Verification items for the finished model (mm, model axes). Face numbers are marked on the shaded views. A direction names the side the tool comes from. Round coordinates to 2 decimals unless told otherwise and drop trailing zeros. Loops run counter-clockwise (first coordinate to the right, second up) from the corner with the lowest first, then second, coordinate; pieces in that order, holes last. Notation, with made-up numbers: (39.5, 80) -> (57.5, 80) arc R11 ccw to (57.5, 91) -> close; hole circle Ø8 at (-29, 84.25). An arc over 180 degrees is marked (long way). Use a Markdown table: item, result. Add a question column.
```python
from build123d import *

# Parameters (mm, degrees)
SKETCH1_W               = 58
SKETCH1_H               = 86
BOSS_EXTRUDE1_DEPTH     = 23
CUT_EXTRUDE1_DEPTH      = 23
CUT_EXTRUDE2_DEPTH      = 23
FILLET1_R               = 3
FILLET2_R               = 2
FILLET3_R               = 2
FILLET4_R               = 1
FILLET5_R               = 3
FILLET6_R               = 3
FILLET7_R               = 3
FILLET8_R               = 3
FILLET9_R               = 3
FILLET10_R              = 3
CUT_EXTRUDE3_DEPTH      = 57.73623181
CUT_EXTRUDE3_DEPTH_BACK = 57.73623181
SKETCH4_W               = 46
SKETCH4_H               = 18
CUT_EXTRUDE4_DEPTH      = 57.73623181
CUT_EXTRUDE4_DEPTH_BACK = 57.73623181
SKETCH5_R               = 2
SKETCH5_R_2             = 1.5
SKETCH6_R               = 1.5
CUT_EXTRUDE11_DEPTH     = 10
SKETCH7_R               = 1.5
CUT_EXTRUDE12_DEPTH     = 10


with BuildPart() as part:
    # Sketch1 → Boss-Extrude1 (new body)
    with BuildSketch(Plane(origin=(0, 0, 0), x_dir=(1, 0, 0), z_dir=(0, 1, 0))):
        Rectangle(SKETCH1_W, SKETCH1_H)
    extrude(amount=BOSS_EXTRUDE1_DEPTH)

    # Sketch2 → Cut-Extrude1 (cut)
    with BuildSketch(Plane(origin=(0, 0, 0), x_dir=(1, 0, 0), z_dir=(0, 1, 0))):
        Polygon((29, -23), (17, -23), (17, -17), (23, -17), (23, -7), (29, -7), align=None)
    extrude(amount=CUT_EXTRUDE1_DEPTH, mode=Mode.SUBTRACT)

    # Sketch3 → Cut-Extrude2 (cut)
    with BuildSketch(Plane(origin=(0, 0, 0), x_dir=(1, 0, 0), z_dir=(0, 1, 0))):
        Polygon((-15, -13), (-15, 22), (18, 22), (18, -1), (6, -1), (6, -13), align=None)
    extrude(amount=CUT_EXTRUDE2_DEPTH, mode=Mode.SUBTRACT)

    # Fillet1
    fillet1_edges = [part.edges().sort_by_distance(p)[0] for p in [
        (23, 11.5, 7),
    ]]
    fillet(fillet1_edges, radius=FILLET1_R)

    # Fillet2
    fillet2_edges = [part.edges().sort_by_distance(p)[0] for p in [
        (17, 11.5, 17),
    ]]
    fillet(fillet2_edges, radius=FILLET2_R)

    # Fillet3
    fillet3_edges = [part.edges().sort_by_distance(p)[0] for p in [
        (17, 11.5, 23),
    ]]
    fillet(fillet3_edges, radius=FILLET3_R)

    # Fillet4
    fillet4_edges = [part.edges().sort_by_distance(p)[0] for p in [
        (23, 11.5, 17),
    ]]
    fillet(fillet4_edges, radius=FILLET4_R)

    # Fillet5
    fillet5_edges = [part.edges().sort_by_distance(p)[0] for p in [
        (-15, 11.5, 13),
    ]]
    fillet(fillet5_edges, radius=FILLET5_R)

    # Fillet6
    fillet6_edges = [part.edges().sort_by_distance(p)[0] for p in [
        (6, 11.5, 13),
    ]]
    fillet(fillet6_edges, radius=FILLET6_R)

    # Fillet7
    fillet7_edges = [part.edges().sort_by_distance(p)[0] for p in [
        (-15, 11.5, -22),
    ]]
    fillet(fillet7_edges, radius=FILLET7_R)

    # Fillet8
    fillet8_edges = [part.edges().sort_by_distance(p)[0] for p in [
        (18, 11.5, -22),
    ]]
    fillet(fillet8_edges, radius=FILLET8_R)

    # Fillet9
    fillet9_edges = [part.edges().sort_by_distance(p)[0] for p in [
        (18, 11.5, 1),
    ]]
    fillet(fillet9_edges, radius=FILLET9_R)

    # Fillet10
    fillet10_edges = [part.edges().sort_by_distance(p)[0] for p in [
        (6, 11.5, 1),
    ]]
    fillet(fillet10_edges, radius=FILLET10_R)

    # Sketch4 → Cut-Extrude3 (cut, two sides: drawn at the far end of the back side and taken through both)
    with BuildSketch(Plane(origin=(0, 0, 0), x_dir=(0, 0, -1), z_dir=(1, 0, 0)).offset(-CUT_EXTRUDE3_DEPTH_BACK)):
        with Locations((0, 9)):
            Rectangle(SKETCH4_W, SKETCH4_H)
    extrude(amount=CUT_EXTRUDE3_DEPTH + CUT_EXTRUDE3_DEPTH_BACK, mode=Mode.SUBTRACT)

    # Sketch5 → Cut-Extrude4 (cut, two sides: drawn at the far end of the back side and taken through both)
    with BuildSketch(Plane(origin=(0, 0, 0), x_dir=(1, 0, 0), z_dir=(0, 1, 0)).offset(-CUT_EXTRUDE4_DEPTH_BACK)):
        with Locations(Location((20.5, -4, 0), (0, 0, 270))):
            Circle(SKETCH5_R)
        with Locations(Location((-20.5, -4, 0), (0, 0, 270))):
            Circle(SKETCH5_R)
        with Locations(Location((20, -14.5, 0), (0, 0, 270))):
            Circle(SKETCH5_R_2)
        with Locations(Location((-16.5, -38, 0), (0, 0, 270))):
            Circle(SKETCH5_R_2)
        with Locations(Location((25.5, -38, 0), (0, 0, 270))):
            Circle(SKETCH5_R_2)
        with Locations(Location((-24.051636808, -28.259079953, 0), (0, 0, 270))):
            Circle(SKETCH5_R_2)
    extrude(amount=CUT_EXTRUDE4_DEPTH + CUT_EXTRUDE4_DEPTH_BACK, mode=Mode.SUBTRACT)

    # Sketch6 → Cut-Extrude11 (cut)
    with BuildSketch(Plane.ZY.offset(29)):
        with Locations((40, 3)):
            Circle(SKETCH6_R)
        with Locations((26, 18)):
            Circle(SKETCH6_R)
    extrude(amount=-CUT_EXTRUDE11_DEPTH, mode=Mode.SUBTRACT)

    # Sketch7 → Cut-Extrude12 (cut)
    with BuildSketch(Plane(origin=(0, 0, -43), x_dir=(-1, 0, 0), z_dir=(0, 0, -1))):
        with Locations((-19.5, 4.5)):
            Circle(SKETCH7_R)
        with Locations((-19.5, 18.5)):
            Circle(SKETCH7_R)
    extrude(amount=-CUT_EXTRUDE12_DEPTH, mode=Mode.SUBTRACT)


solid = part.part
```
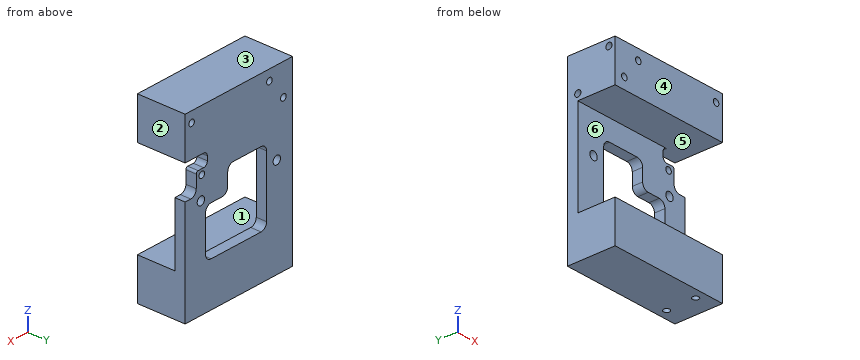
1) Sectioned sample at D-D on x = -5. Enter the section's corners in (y, z).
2) Sectioned sample at B-B on y = 15.5. Enter the section's corners in (x, z).
3) Access from +Z, -Z, +X, -X, +Y, -Y to the whole of each face (thin tool, end or side, straight path). Record for the marked faces 1 and 2.
4) Sectioned sample at C-C on z = 14.5. Enter the section's corners in (x, y), then the cut area to 3 significant figures.
5) Go/stop test with flat-tipped pins: pin 1 (2.5 mm diameter, centred on x = -16.5, z = 38, fed in from -Y); pin 2 (1.5 mm diameter, centred on y = 3.5, z = 40, fed in from -X); pin 3 (2.5 mm diameter, centred on x = 19.5, y = 4.5, fed in from -Z); pin 4 (23 mm diameter, centred on x = 13, z = -8, fed in from -Y). Record where each tip stops, or that it passes through.
6) Thickness scan on line 1 (X direction, y = 16.5, z = 38); line 2 (X direction, y = 20.2, z = 4); line 3 (Y direction, x = 19.5, z = -36). Record the ranges inside material, lowest first.
7) Sectioned sample at A-A on x = -16.5. Enter the section's corners in (y, z).
8) Release check for a two-part mould opening along Z. For the marked faces 3, 4, 5 and 6 record: released by +Z, released by -Z, zero draft, split by the parting line, or undercut.
Geometry results:
| question | item | result |
|---|---|---|
| 1 | outline | (0, -43) -> (23, -43) -> (23, -22) -> (18, -22) -> (18, -23) -> (0, -23) -> close; (0, 23) -> (18, 23) -> (18, 13) -> (23, 13) -> (23, 43) -> (0, 43) -> close |
| 2 | outline | (-29, -43) -> (29, -43) -> (29, -23) -> (-29, -23) -> close; (-29, 23) -> (29, 23) -> (29, 43) -> (-29, 43) -> close; hole circle Ø3 at (-24.05, 28.26); hole circle Ø3 at (-16.5, 38); hole circle Ø3 at (25.5, 38) |
| 3 | face 1 | +X, -X, -Y |
| 3 | face 2 | +Z, -Z, +X, +Y, -Y |
| 4 | outline | (-29, 18) -> (18.5, 18) -> (18.5, 23) -> (-29, 23) -> close; (21.5, 18) -> (23, 18) -> (23, 23) -> (21.5, 23) -> close |
| 4 | area | 245 mm^2 |
| 5 | pin 1 | through |
| 5 | pin 2 | x = -19 |
| 5 | pin 3 | z = -33 |
| 5 | pin 4 | y = 18 |
| 6 | line 1 | -29 to -18, -15 to 24, 27 to 29 |
| 6 | line 2 | -29 to -22.5, -18.5 to -15, 6 to 18.5, 22.5 to 29 |
| 6 | line 3 | 0 to 3, 6 to 17, 20 to 23 |
| 7 | outline | (0, -43) -> (23, -43) -> (23, 36.5) -> (0, 36.5) -> (0, 23) -> (18, 23) -> (18, -23) -> (0, -23) -> close; (0, 39.5) -> (23, 39.5) -> (23, 43) -> (0, 43) -> close |
| 8 | face 3 | released by +Z |
| 8 | face 4 | zero draft |
| 8 | face 5 | undercut |
| 8 | face 6 | undercut |
